Work out the finished part from the listing and answer in its coordinate system (mm). Face numbers are marked on the shaded views. Give positions to 0.01 mm unless a question says otherwise; leave off trailing zeros. Loops run counter-clockwise (first coordinate to the right, second up) from the corner with the lowest first, then second, coordinate; pieces in that order, holes last.
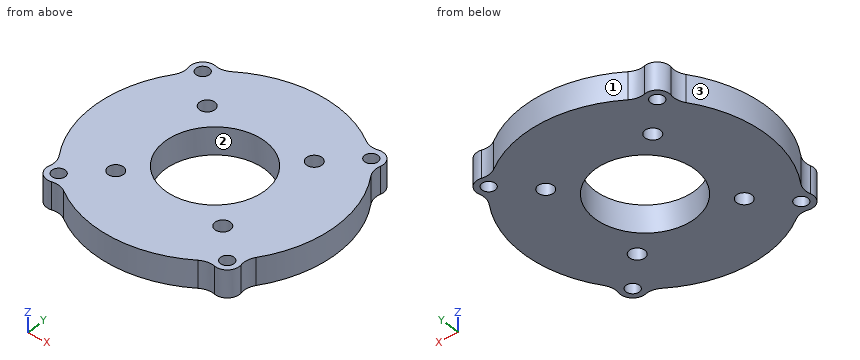
Autodesk Inventor part; units mm, degrees
ref_plane "YZ Plane" through (0, 0, 0) normal (1, 0, 0) x (0, 1, 0)
ref_plane "XZ Plane" through (0, 0, 0) normal (0, 1, 0) x (-1, 0, 0)
ref_plane "XY Plane" through (0, 0, 0) normal (0, 0, 1) x (1, 0, 0)
sketch "Base" plane through (0, 0, 0) normal (0, 0, 1) x (1, 0, 0)
  circle A0 centre (0, 0) radius 50.8
  circle A1 centre (0, 0) radius 16.5
  line L0 (-71.12, 0) -> (71.12, 0)
  line L1 (0, -71.12) -> (0, 71.12) construction
  circle A2 centre (-17.9605, 17.9605) radius 2.5527
  circle A3 centre (17.9605, 17.9605) radius 2.5527
  circle A4 centre (17.9605, -17.9605) radius 2.5527
  circle A5 centre (-17.9605, -17.9605) radius 2.5527
  circle A6 centre (0, 0) radius 16 construction
  circle A7 centre (0, 0) radius 40
  line L2 (0, 0) -> (28.2843, 28.2843) construction
  circle A8 centre (28.2843, 28.2843) radius 2.2
  circle A9 centre (-28.2843, 28.2843) radius 2.2
  circle A10 centre (28.2843, -28.2843) radius 2.2
  circle A11 centre (-28.2843, -28.2843) radius 2.2
  circle A12 centre (28.2843, 28.2843) radius 4
  circle A13 centre (17.9605, 17.9605) radius 4
  circle A14 centre (-17.9605, 17.9605) radius 4
  circle A15 centre (-28.2843, 28.2843) radius 4
  line L3 (0, 0) -> (35.921, 35.921)
  line L4 (0, 0) -> (-35.921, 35.921)
  circle A16 centre (28.2843, -28.2843) radius 4
  circle A17 centre (-28.2843, -28.2843) radius 4
  circle A18 centre (17.9605, -17.9605) radius 4
  circle A19 centre (-17.9605, -17.9605) radius 4
  point P0 (-25.4558, 25.4558)
  point P1 (-20.7889, 20.7889)
  point P2 (-15.1321, 15.1321)
  point P3 (-11.6673, 11.6673)
  point P4 (11.6673, 11.6673)
  point P5 (15.1321, 15.1321)
  point P6 (20.7889, 20.7889)
  point P7 (25.4558, 25.4558)
  point P8 (31.1127, 31.1127)
  point P9 (-31.1127, 31.1127)
  point P10 (25.318, 30.9677)
  point P11 (-25.318, 30.9677)
  point P12 (-30.9677, 25.318)
  point P13 (-40, 0)
  point P14 (-16.5, 0)
  point P15 (16.5, 0)
  point P16 (40, 0)
  point P17 (30.9677, 25.318)
  point P18 (30.9677, -25.318)
  point P19 (-30.9677, -25.318)
  point P20 (-25.318, -30.9677)
  point P21 (25.318, -30.9677)
  dimension "d26" = 80
  dimension "d0" = 101.6
  dimension "d25" = 0.5
  dimension "d27" = 4.4
  dimension "d29" = 8
extrude "Plate1" add sketch "Base" along normal blind 9 contours A7 A16 A17 L0 A1 | L0 A1 L3 A13 A12 A7 | L3 A8 A7 A12 | A12 A7 A8 L3 | A7 A15 L4 A14 A1 L0 | A12 L3 A8 A7 | A16 A7 A10 | A7 A10 A16 | L4 A9 A7 A15 | A15 A7 A9 L4 | A12 L3 A13 A1 L4 A14 A15 A7 | A7 A8 L3 A12 | A7 A9 L4 A15 | A17 A7 A11 | A7 A11 A17 | A15 L4 A9 A7 | L3 A3 A13 | A13 L3 A3 | L4 A2 A14 | A14 L4 A2 | A18 | A19
fillet "Fillet2" radius 6 8 edges at (-30.9677, 25.318, 4.5) (-30.9677, -25.318, 4.5) (-25.318, -30.9677, 4.5) (25.318, -30.9677, 4.5) (30.9677, -25.318, 4.5) (30.9677, 25.318, 4.5) (25.318, 30.9677, 4.5) (-25.318, 30.9677, 4.5)
equation "\"d28\" = Thickness"
equation "\"BendRadius\" = Thickness"
equation "\"BendReliefWidth\" = Thickness"
equation "\"BendReliefDepth\" = 0.5 * Thickness"
equation "\"CornerReliefSize\" = 4 * Thickness"
equation "\"MinimumRemnant\" = 2 * Thickness"
equation "\"TransitionRadius\" = BendRadius"
equation "\"JacobiRadiusSize\" = BendRadius"
equation "\"GapSize\" = Thickness"
properties part number "CimCoderMount"
Item 1: Find section D-D, the plane y = 19. Write down the section's boundary in (x, z).
Item 2: Find section A-A, the plane x = 0. Write down the section's boundary in (y, z).
Item 3: Find section B-B, the plane y = -12. Write down the section's boundary in (x, z).
Item 4: Find section C-C, the plane x = 17.5. Write down the section's boundary in (y, z).
Item 5: Consider line 1 (X direction, y = 28.5, z = 2.75); line 2 (Y direction, x = 27.5, z = 8); line 3 (X direction, y = -18.5, z = 1). Determine where each line is inside the solid, lowest interval first.
Item 6: Flat-ended cylindrical pins translate along their axes: pin 1 Ø3 at (y, z) = (-1.5, 6) entering from +X; pin 2 Ø1.5 at (x, z) = (19.5, 6.5) entering from +Y; pin 3 Ø4 at (x, z) = (14, 8) entering from +Y; pin 4 Ø3 at (x, z) = (-3, 5) entering from +Y. Find the tip coordinate at first contact, or state that the pin passes through.
Item 7: Determine the mould class of the marked faces 1, 2 and 3 for opening direction X: released by +X, released by -X, zero draft, split by the parting line, or undercut.
Ans:
1. outline: (-35.2, 0) - (-20.29, 0) - (-20.29, 9) - (-35.2, 9) - close; (-15.63, 0) - (15.63, 0) - (15.63, 9) - (-15.63, 9) - close; (20.29, 0) - (35.2, 0) - (35.2, 9) - (20.29, 9) - close
2. outline: (-40, 0) - (-16.5, 0) - (-16.5, 9) - (-40, 9) - close; (16.5, 0) - (40, 0) - (40, 9) - (16.5, 9) - close
3. outline: (-38.16, 0) - (-11.32, 0) - (-11.32, 9) - (-38.16, 9) - close; (11.32, 0) - (38.16, 0) - (38.16, 9) - (11.32, 9) - close
4. outline: (-35.97, 0) - (-20.47, 0) - (-20.47, 9) - (-35.97, 9) - close; (-15.45, 0) - (15.45, 0) - (15.45, 9) - (-15.45, 9) - close; (20.47, 0) - (35.97, 0) - (35.97, 9) - (20.47, 9) - close
5. line 1: x = -32.28 to -30.47, -26.09 to 26.09, 30.47 to 32.28
5. line 2: y = -32.21 to -30.34, -26.23 to 26.23, 30.34 to 32.21
5. line 3: x = -35.46 to -20.46, -15.47 to 15.47, 20.46 to 35.46
6. pin 1: stops at x = 40
6. pin 2: stops at y = 35.33
6. pin 3: stops at y = 38.16
6. pin 4: stops at y = 39.97
7. face 1: split by the parting line
7. face 2: undercut
7. face 3: released by -X
